Read the model definition and answer for the solid it produces. Units are mm, in the model's axes. A direction names the side the tool comes from. Coordinates: 2 decimals unless noted, no trailing zeros. Write each loop counter-clockwise with the first axis right and the second up, starting at its lowest first coordinate (ties: lowest second). Pieces come first, ordered by that corner, then holes. Notation, with made-up numbers: (-2.5, 18) -> (5.5, 18) arc R26 ccw to (5.5, 43) -> close; hole circle Ø10 at (8.5, 15). An arc over 180 degrees is marked (long way). Write item = value, one per line. Start each with the question number.
1) A tool of negligible diameter and unlimited length cuts with its end or side. For faces 1 (the face through (-7.509, 33.734, -23.846)), 2 (the face through (7.91, 64.698, 10.316)), from which of +Z, -Z, +X, -X, +Y, -Y can it reach the whole face along a straight path? Write none if from no direction.
2) Section B-B (x = 0) is taken. Determine the outline of the cut face in (y, z).
3) Find the intervals of material crossed by line 1 along X through (y, z) = (45.5, 0); line 2 along Z through (x, y) = (2, 65); line 3 along Z through (x, y) = (-0.5, 55.5), in increasing order. Write a range as from..to.
4) Section D-D (y = 24) is taken. Determine the outline of the cut face in (x, z).
5) Section A-A (z = 0) is taken. Determine the outline of the cut face in (x, y).
6) For a pull along Z with two mould halves and no side action, classify faces 3 (the face through (8.88, 4.06, -21.41)), 4 (the face through (5, 0, 0)), 5 (the face through (0.9, 34.73, 2.86)) as released by +Z, released by -Z, zero draft, split by the parting line, or undercut.
7) Flat-ended cylindrical pins translate along their axes: pin 1 Ø6 at (x, z) = (-16, -14) entering from +Y; pin 2 Ø1.5 at (y, z) = (54, -1.5) entering from +X; pin 3 Ø1 at (x, y) = (14.5, 23) entering from -Z. Find the tip coordinate at first contact, or state that the pin passes through.
8) Section C-C (y = 54.5) is taken. Determine the outline of the cut face in (x, z), plus the area to 3 significant figures.
from build123d import *

# Parameters (mm, degrees)
SKETCH2_R          = 3
CUT_EXTRUDE1_DEPTH = 70


with BuildPart() as part:
    # Sketch1 → Revolve1 (revolve)
    with BuildSketch(Plane.XY, mode=Mode.PRIVATE) as revolve1_sk:
        Polygon((22.5, 0), (0, 0), (0, 68.5), (13, 68.5), (13, 61), (25, 53), (25, 15), align=None)
    revolve(revolve1_sk.sketch.rotate(Axis((0, 0, 0), (0, 1, 0)), 90), axis=Axis((0, 0, 0), (0, 1, 0)))

    # Sketch2 → Cut-Extrude1 (cut)
    with BuildSketch(Plane(origin=(0, 68.5, 0), x_dir=(1, 0, 0), z_dir=(0, 1, 0))):
        with Locations(Location((0, 0, 0), (0, 0, 270))):
            Circle(SKETCH2_R)
    extrude(amount=-CUT_EXTRUDE1_DEPTH, mode=Mode.SUBTRACT)


solid = part.part
Answer key:
q1.face_1 = +Y, -Y
q1.face_2 = +Y
q2.outline = (0, -22.5) -> (15, -25) -> (53, -25) -> (61, -13) -> (68.5, -13) -> (68.5, -3) -> (0, -3) -> close; (0, 3) -> (68.5, 3) -> (68.5, 13) -> (61, 13) -> (53, 25) -> (15, 25) -> (0, 22.5) -> close
q3.line_1 = -25..-3, 3..25
q3.line_2 = -12.85..-2.24, 2.24..12.85
q3.line_3 = -21.24..-2.96, 2.96..21.24
q4.outline = circle Ø50 at (0, 0); hole circle Ø6 at (0, 0)
q5.outline = (-25, 15) -> (-22.5, 0) -> (-3, 0) -> (-3, 68.5) -> (-13, 68.5) -> (-13, 61) -> (-25, 53) -> close; (3, 0) -> (22.5, 0) -> (25, 15) -> (25, 53) -> (13, 61) -> (13, 68.5) -> (3, 68.5) -> close
q6.face_3 = split by the parting line
q6.face_4 = zero draft
q6.face_5 = undercut
q7.pin_1 = 57.49
q7.pin_2 = 24.58
q7.pin_3 = -20.71
q8.outline = circle Ø45.5 at (0, 0); hole circle Ø6 at (0, 0)
q8.area = 1,600 mm^2
